```python
from build123d import *

# Parameters (mm, degrees)
F0_W     = 40
F0_H     = 40
F0_W_2   = 34.8
F0_H_2   = 34.8
F1_DEPTH = 576
F2_R     = 4
F3_R     = 2


with BuildPart() as f1:
    # F0 (on Front) → F1 (new body)
    with BuildSketch(Plane.XZ):
        Rectangle(F0_W, F0_H)
        Rectangle(F0_W_2, F0_H_2, mode=Mode.SUBTRACT)
    extrude(amount=F1_DEPTH)

    # F2
    f2_edges = [f1.edges().sort_by_distance(p)[0] for p in [
        (20, -288, 20),
        (-20, -288, 20),
        (20, -288, -20),
        (-20, -288, -20),
    ]]
    fillet(f2_edges, radius=F2_R)

    # F3
    f3_edges = [f1.edges().sort_by_distance(p)[0] for p in [
        (-17.4, -288, 17.4),
        (-17.4, -288, -17.4),
        (17.4, -288, -17.4),
        (17.4, -288, 17.4),
    ]]
    fillet(f3_edges, radius=F3_R)


solid = f1.part
```
For this review, take the finished solid that the model builds, in its own axes (mm). A direction names the side the tool comes from. Coordinates: 2 decimals unless noted, no trailing zeros. Loops run counter-clockwise (first coordinate to the right, second up) from the corner with the lowest first, then second, coordinate; pieces in that order, holes last. Notation, with made-up numbers: (-28.5, 24.5) - (-1.5, 24.5) arc R20 ccw to (-1.5, 60.5) - close; hole circle Ø1 at (21, 74). An arc over 180 degrees is marked (long way). Use one line per item in the form item = value. Start each with the question number.
1) Draft analysis for pull direction X (two halves, no side actions). For faces 3 (the face through (0, -284, 20)), 4 (the face through (-20, -284, 0)), 5 (the face through (-17.4, -284, 0)), 6 (the face through (0, -284, -17.4)), state which applies: released by +X, released by -X, zero draft, split by the parting line, or undercut.
2) For faces 1 (the face through (-18, -576, 0)), 2 (the face through (17.4, -284, 0)), list the 3-axis set-ups (+Z, -Z, +X, -X, +Y, -Y) from which the entire face can be reached by the end or side of a thin tool; tool diameter is ignored.
3) To check wall thickness, follow probe 1 along Z at (x, y) = (8.5, -264.5); probe 2 along X at (y, z) = (-63.5, -17). State the ranges of each line that lie inside material, in increasing order. Write a range as from..to.
4) For pin 1 (2 mm diameter, centred on x = -3.5, z = -15, fed in from +Y), flat-tipped, find the tip position at first contact; note if it passes through.
5) Take a section at C-C (y = -289). State the section outline as (x, z) points.
6) Take a section at B-B (x = 9.5). State the section outline as (y, z) points, plus the area to 3 significant figures.
7) Take a section at A-A (z = -5.5). State the section outline as (x, y) points.
From the geometry:
q1.face_3 = zero draft
q1.face_4 = released by -X
q1.face_5 = undercut
q1.face_6 = undercut
q2.face_1 = +Z, -Z, +X, -X, -Y
q2.face_2 = +Y, -Y
q3.probe_1 = -20..-17.4, 17.4..20
q3.probe_2 = -19.87..-16.6, 16.6..19.87
q4.pin_1 = through
q5.outline = (-20, -16) arc R4 ccw to (-16, -20) - (16, -20) arc R4 ccw to (20, -16) - (20, 16) arc R4 ccw to (16, 20) - (-16, 20) arc R4 ccw to (-20, 16) - close; hole (-17.4, -15.4) arc R2 ccw to (-15.4, -17.4) - (15.4, -17.4) arc R2 ccw to (17.4, -15.4) - (17.4, 15.4) arc R2 ccw to (15.4, 17.4) - (-15.4, 17.4) arc R2 ccw to (-17.4, 15.4) - close
q6.outline = (-576, -20) - (0, -20) - (0, -17.4) - (-576, -17.4) - close; (-576, 17.4) - (0, 17.4) - (0, 20) - (-576, 20) - close
q6.area = 3,000 mm2
q7.outline = (-20, -576) - (-17.4, -576) - (-17.4, 0) - (-20, 0) - close; (17.4, -576) - (20, -576) - (20, 0) - (17.4, 0) - close
